Read the model definition and answer for the solid it produces. Units are mm, in the model's axes. Coordinates: 2 decimals unless noted, no trailing zeros. Loops run counter-clockwise (first coordinate to the right, second up) from the corner with the lowest first, then second, coordinate; pieces in that order, holes last. Notation, with made-up numbers: (25.5, 71) -> (45.5, 71) arc R13 cw to (45.5, 77) -> close; hole circle Ø9 at (51.5, 81). An arc over 180 degrees is marked (long way). One line per question, with ' | ' between items. Start each with the question number.
```python
from build123d import *

# Parameters (mm, degrees)
F0_W     = 24.73539114
F0_H     = 419.7955727577
F2_DEPTH = 425.6457388401
F3_SIZE  = 22.86
F4_SIZE  = 5.08
F5_SIZE  = 2.54


with BuildPart() as f1:
    # F0 (on Front) → F1 (revolve)
    with BuildSketch(Plane.XZ):
        with Locations((-12.36769557, -30.4397642612)):
            Rectangle(F0_W, F0_H)
    revolve(axis=Axis((0, 0, -30.4397642612), (0, 0, -1)))

    # F2 (add): a face of the model
    f2_faces = [f1.faces().sort_by_distance(p)[0] for p in [
        (0, 0, -240.3375506401),
    ]]
    extrude(f2_faces, amount=F2_DEPTH)

    # F3
    f3_edges = [f1.edges().sort_by_distance(p)[0] for p in [
        (24.735391, 0, -665.983289),
    ]]
    chamfer(f3_edges, length=F3_SIZE)

    # F4
    f4_edges = [f1.edges().sort_by_distance(p)[0] for p in [
        (24.735391, 0, -643.123289),
    ]]
    chamfer(f4_edges, length=F4_SIZE)

    # F5
    f5_edges = [f1.edges().sort_by_distance(p)[0] for p in [
        (24.735385, 0, -638.043289),
    ]]
    chamfer(f5_edges, length=F5_SIZE)


solid = f1.part
```
(1) Section A-A on z = 57.5 is taken. Write down the section's boundary in (x, y).
(2) Find the intervals of material crossed by probe 1 along Y at (x, z) = (-2, 46); probe 2 along Y at (x, z) = (-13, -445); probe 3 along X at (y, z) = (-1.5, -29), in increasing order. Write a range as from..to.
(3) Each of these flat-tipped pins is pushed along its axis until it touches: pin 1 Ø4 at (x, y) = (13, 13) entering from -Z; pin 2 Ø8 at (y, z) = (-0.5, -578) entering from +X; pin 3 Ø4 at (y, z) = (-10, -302.5) entering from -X; pin 4 Ø1.5 at (x, z) = (-2.5, -85.5) entering from +Y. Where does it stop, or does it pass through?
Working result:
1) outline: circle Ø49.47 at (0, 0)
2) probe 1: y = -24.65..24.65 | probe 2: y = -21.04..21.04 | probe 3: x = -24.69..24.69
3) pin 1: stops at z = -651.47 | pin 2: stops at x = 24.74 | pin 3: stops at x = -23.41 | pin 4: stops at y = 24.67
